Input: dimensioned drawing with shaded views. Units: mm. Origin: part minimum x, y, z. A direction names the side the tool comes from. Give positions to 0.01 mm unless a question says otherwise; leave off trailing zeros. Loops run counter-clockwise (first coordinate to the right, second up) from the corner with the lowest first, then second, coordinate; pieces in that order, holes last.
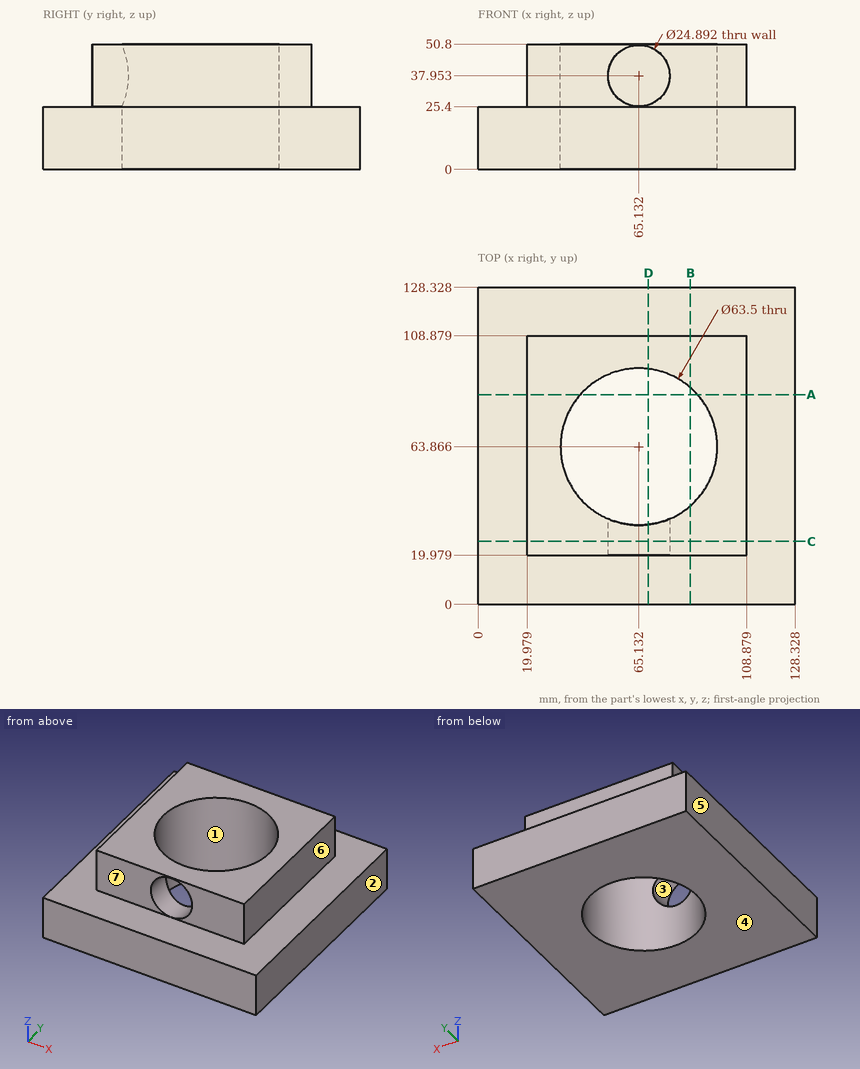
Item 1: Section query B-B on x = 86. Return loops of the section in (y, z) (1 decimal).
Values follow:
outline: (0, 0) - (39.9, 0) - (39.9, 50.8) - (20, 50.8) - (20, 25.4) - (0, 25.4) - close; (87.8, 0) - (128.3, 0) - (128.3, 25.4) - (108.9, 25.4) - (108.9, 50.8) - (87.8, 50.8) - close
Item 2: Ray query, probe 1 along Z at (x, y) = (56.5, 12); probe 2 along X at (y, z) = (105, 34.5); probe 3 along Y at (x, z) = (45, 24.5) (1 decimal). Return the intervals inside material, ascending.
Values follow:
probe 1: z = 0 to 25.4
probe 2: x = 19.98 to 108.88
probe 3: y = 0 to 39.3, 88.4 to 128.3
Item 3: Pin query (flat end, axial travel): pin 1 (22.5 mm diameter, centred on x = 65.13, z = 37.95, fed in from -Y) (1 decimal); pin 2 (4 mm diameter, centred on y = 104.5, z = 33.5, fed in from -X); pin 3 (6 mm diameter, centred on y = 111.5, z = 34, fed in from +X). Return the tip coordinate at first contact, or that it passes through.
Values follow:
pin 1: stops at y = 93.6
pin 2: stops at x = 19.98
pin 3: stops at x = 108.88
Item 4: Draft query along X for the marked faces 1, 2, 3 and 4. Return one class per face: +X half, -X half, draft (parallel to the pull), parting line (faces both ways), or undercut.
Values follow:
face 1: undercut
face 2: +X half
face 3: undercut
face 4: draft
Item 5: Set-up query: the marked faces 5, 6 and 7. Return all of +Z, -Z, +X, -X, +Y, -Y with unobstructed straight access to the full face (end or side cutting, diameter ignored); none if empty.
Values follow:
face 5: +Z, -Z, -X, +Y, -Y
face 6: +Z, +X, +Y, -Y
face 7: +Z, +X, -X, -Y
Item 6: Section query C-C on y = 25.5. Return loops of the section in (x, z).
Values follow:
outline: (0, 0) - (128.33, 0) - (128.33, 25.4) - (108.88, 25.4) - (108.88, 50.8) - (19.98, 50.8) - (19.98, 25.4) - (0, 25.4) - close; hole circle Ø24.89 at (65.13, 37.95)
Item 7: Section query D-D on x = 69. Return loops of the section in (y, z).
Values follow:
outline: (0, 0) - (32.35, 0) - (32.35, 26.12) - (19.98, 26.12) - (19.98, 25.4) - (0, 25.4) - close; (19.98, 49.78) - (32.35, 49.78) - (32.35, 50.8) - (19.98, 50.8) - close; (95.38, 0) - (128.33, 0) - (128.33, 25.4) - (108.88, 25.4) - (108.88, 50.8) - (95.38, 50.8) - close
Item 8: Section query A-A on y = 85. Return loops of the section in (x, z).
Values follow:
outline: (0, 0) - (41.44, 0) - (41.44, 50.8) - (19.98, 50.8) - (19.98, 25.4) - (0, 25.4) - close; (88.83, 0) - (128.33, 0) - (128.33, 25.4) - (108.88, 25.4) - (108.88, 50.8) - (88.83, 50.8) - close
